```python
from build123d import *

# Parameters (mm, degrees)
ESBO_O1_W                = 4
ESBO_O1_H                = 7
RESSALTO_EXTRUS_O1_DEPTH = 5
FILETE1_R                = 2
ESBO_O4_W                = 2
ESBO_O4_H                = 1
CORTE_EXTRUS_O2_DEPTH    = 12


with BuildPart() as part:
    # Esboço1 → Ressalto-extrusão1 (new body)
    with BuildSketch(Plane.XY):
        Polygon((24, 3.5), (24, 6.5), (12, 6.5), (12, 10), (0, 10), (0, 0), (12, 0), (12, 3.5), align=None)
        with Locations((6, 5)):
            Rectangle(ESBO_O1_W, ESBO_O1_H, mode=Mode.SUBTRACT)
    extrude(amount=RESSALTO_EXTRUS_O1_DEPTH)

    # Filete1
    filete1_edges = [part.edges().sort_by_distance(p)[0] for p in [
        (8, 5, 5),
    ]]
    fillet(filete1_edges, radius=FILETE1_R)

    # Esboço4 → Corte-extrusão2 (cut)
    with BuildSketch(Plane(origin=(24, 0, 0), x_dir=(0, 0, -1), z_dir=(1, 0, 0))):
        with Locations((-1, 4)):
            Rectangle(ESBO_O4_W, ESBO_O4_H)
        with Locations((-1, 6)):
            Rectangle(ESBO_O4_W, ESBO_O4_H)
    extrude(amount=-CORTE_EXTRUS_O2_DEPTH, mode=Mode.SUBTRACT)


solid = part.part
```
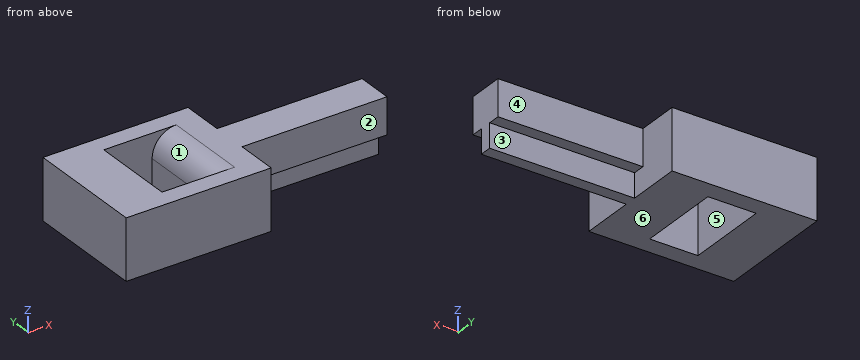
Geometry check sheet. Reference: the model listing, model coordinates, mm. Face numbers are marked on the shaded views. A direction names the side the tool comes from. Round coordinates to 2 decimals unless told otherwise and drop trailing zeros. Order: outer loops, then holes, each group sorted by start corner. A loop starts at its lowest first (then second) coordinate and runs counter-clockwise, first axis right, second up. Notation, with made-up numbers: M -16.75,-11.75 L 39.25,-11.75 A7 ccw 39.25,0.25 Z; hole C 20.25,83 d1. An arc over 180 degrees is marked long. Write item = value, one per line.
Q1. Set-up check for the marked faces 4, 5 and 6: record each of +Z, -Z, +X, -X, +Y, -Y from which the full face is reachable in a straight line by a thin tool's end or side.
Answer block:
face_4 = +Z, -Z, +X, +Y
face_5 = +Z, -Z
face_6 = -Z, +X, -X, +Y, -Y
Q2. Depth check by flat-ended pin: pin 1 Ø2 at (x, z) = (16, 0.5) entering from +Y; pin 2 Ø1.5 at (x, z) = (15, 3) entering from +Y; pin 3 Ø1.5 at (x, z) = (15.5, 3) entering from -Y. Enter the tip coordinate at first touch or a pass-through.
Answer block:
pin_1 = 5.5
pin_2 = 6.5
pin_3 = 3.5
Q3. Scan lines: line 1 (X direction, y = 1.75, z = 1.8); line 2 (Y direction, x = 7.5, z = 3.5); line 3 (X direction, y = 5, z = 1.2). Record each from-to range of solid material in increasing order.
Answer block:
line_1 = 0 to 4, 8 to 12
line_2 = 0 to 1.5, 8.5 to 10
line_3 = 0 to 4, 8 to 24
Q4. Section check A-A (y = 6.25). Enter the section's corners in (x, z), plus the area to 3 significant figures.
Answer block:
outline = M 0,0 L 4,0 L 4,5 L 0,5 Z; M 8,0 L 12,0 L 12,2 L 24,2 L 24,5 L 10,5 A2 ccw 8,3 Z
area = 75.1 mm^2
Q5. Section check C-C (z = 1.7). Enter the section's corners in (x, y), plus the area to 3 significant figures.
Answer block:
outline = M 0,0 L 12,0 L 12,4.5 L 24,4.5 L 24,5.5 L 12,5.5 L 12,10 L 0,10 Z; hole M 4,1.5 L 8,1.5 L 8,8.5 L 4,8.5 Z
area = 104 mm^2
Q6. Section check B-B (x = 5). Enter the section's corners in (y, z).
Answer block:
outline = M 0,0 L 1.5,0 L 1.5,5 L 0,5 Z; M 8.5,0 L 10,0 L 10,5 L 8.5,5 Z
Q7. Section check D-D (x = 20). Enter the section's corners in (y, z).
Answer block:
outline = M 3.5,2 L 4.5,2 L 4.5,0 L 5.5,0 L 5.5,2 L 6.5,2 L 6.5,5 L 3.5,5 Z
Q8. Release check for a two-part mould opening along Y. For the marked faces 1, 2 and 3 record: released by +Y, released by -Y, zero draft, split by the parting line, or undercut.
Answer block:
face_1 = undercut
face_2 = released by -Y
face_3 = released by +Y
